Read the model definition and answer for the solid it produces. Units are mm, in the model's axes. Face numbers are marked on the shaded views. A direction names the side the tool comes from. Round coordinates to 2 decimals unless told otherwise and drop trailing zeros. Order: outer loops, then holes, each group sorted by start corner. A loop starts at its lowest first (then second) coordinate and runs counter-clockwise, first axis right, second up.
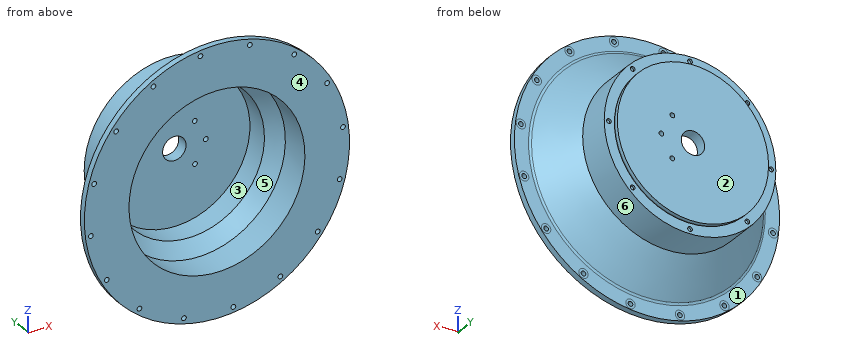
from build123d import *
from build123d.topology import SkipClean

# Parameters (mm, degrees)
SKETCH_1_R               = 85
EXTRUDE_1_DEPTH          = 4
SKETCH_2_R               = 56.4
CUT_EXTRUDE_1_DEPTH      = 50
EXTRUDE_2_REACH          = 125.657
SKETCH_8_R               = 68.956948121
SKETCH_8_R_2             = 56.4
SKETCH_9_R               = 1.5
CUT_EXTRUDE_3_DEPTH      = 5000
PATTERN_CIRCULAR_1_COUNT = 16
SKETCH_11_R              = 52.5
SKETCH_11_R_2            = 48.463912786
EXTRUDE_3_DEPTH          = 30
SKETCH_12_R              = 52.5
SKETCH_12_R_2            = 22.5
EXTRUDE_4_DEPTH          = 5
FILLET_1_R               = 2
SKETCH_13_R              = 85
SKETCH_13_R_2            = 56.4
EXTRUDE_5_DEPTH          = 1
SKETCH_14_R              = 1.5
CUT_EXTRUDE_4_DEPTH      = 50
PATTERN_CIRCULAR_2_COUNT = 16
CHAMFER_2_SIZE           = 5
SKETCH_15_R              = 45
SKETCH_15_R_2            = 43
CUT_EXTRUDE_5_DEPTH      = 2
EXTRUDE_START            = -5
SKETCH_16_R              = 22.5
SKETCH_16_R_2            = 15
EXTRUDE_6_DEPTH          = 5
SKETCH_18_R              = 3
CUT_EXTRUDE_7_DEPTH      = 0.002
PATTERN_CIRCULAR_3_COUNT = 16
EXTRUDE_7_REACH          = 138.657
SKETCH_19_R              = 55
SKETCH_19_R_2            = 49.128121992
SKETCH_20_R              = 47.909164775
SKETCH_20_R_2            = 36.467922282
EXTRUDE_9_DEPTH          = 2
SKETCH_21_R              = 61.010488539
CUT_EXTRUDE_8_DEPTH      = 15
SKETCH_22_R              = 55
EXTRUDE_11_DEPTH         = 5
SKETCH_23_R              = 1.5
CUT_EXTRUDE_9_DEPTH      = 2
PATTERN_CIRCULAR_4_COUNT = 8
SKETCH_24_R              = 48.5
EXTRUDE_12_DEPTH         = 3
SKETCH_25_R              = 7.5
CUT_EXTRUDE_10_DEPTH     = 500
SKETCH_26_R              = 99.377055334
CUT_EXTRUDE_11_DEPTH     = 1
SKETCH_27_R              = 55
SKETCH_27_R_2            = 48.5
CUT_EXTRUDE_13_DEPTH     = 0.5
SKETCH_28_R              = 50.330006294
CUT_EXTRUDE_14_DEPTH     = 0.5
SKETCH_17_R              = 1.5
CUT_EXTRUDE_17_DEPTH     = 20


with BuildPart() as part:
    # 草图1 → 凸台-拉伸1 (new body)
    with BuildSketch(Plane(origin=(0, 0, 0), x_dir=(1, 0, 0), z_dir=(0, 1, 0))):
        with Locations(Location((0, 0, 0), (0, 0, 270))):
            Circle(SKETCH_1_R)
    extrude(amount=EXTRUDE_1_DEPTH)

    # 草图2 → 切除-拉伸1 (cut)
    with BuildSketch(Plane(origin=(0, 4, 0), x_dir=(1, 0, 0), z_dir=(0, 1, 0))):
        with Locations(Location((0, 0, 0), (0, 0, 270))):
            Circle(SKETCH_2_R)
    extrude(amount=-CUT_EXTRUDE_1_DEPTH, mode=Mode.SUBTRACT)

    # 草图3 → 旋转1 (revolve)
    with BuildSketch(Plane.XY):
        Polygon((0, 4), (-75, 4), (-52.5, 29), (0, 29), align=None)
    revolve(axis=Axis((0, 29, 0), (0, -1, 0)))

    # 草图7 → 切除-旋转1 (revolve, cut)
    with BuildSketch(Plane.XY, mode=Mode.PRIVATE) as cut_revolve_1_sk:
        Polygon((0, 4), (-70.963912786, 4), (-48.463912786, 29), (0, 29), align=None)
    revolve(cut_revolve_1_sk.sketch.rotate(Axis((0, 29, 0), (0, -1, 0)), 270), axis=Axis((0, 29, 0), (0, -1, 0)), mode=Mode.SUBTRACT)

    # 凸台-拉伸2: up to this cone (the profile starts inside it)
    extrude_2_end = Plane(origin=(0, 0, 0), z_dir=(0, -1, 0)).offset(-82.848790984) * Cone(1e-06, 255.212734293, 283.56970377, align=(Align.CENTER, Align.CENTER, Align.MIN), mode=Mode.PRIVATE)
    # 草图8 → 凸台-拉伸2 (add, up to the surface)
    with BuildSketch(Plane.XZ, mode=Mode.PRIVATE) as extrude_2_sk1:
        with Locations(Location((0, 0, 0), (0, 0, 270))):
            Circle(SKETCH_8_R)
        with Locations(Location((0, 0, 0), (0, 0, 90))):
            Circle(SKETCH_8_R_2, mode=Mode.SUBTRACT)
    extrude_2_tool1 = extrude(extrude_2_sk1.sketch, amount=-EXTRUDE_2_REACH, mode=Mode.PRIVATE) & extrude_2_end
    add(extrude_2_tool1.solids().sort_by_distance((0, 0, 67.006551))[0])

    # 草图9 → 切除-拉伸3 (cut)
    with BuildSketch(Plane(origin=(0, 4, 0), x_dir=(1, 0, 0), z_dir=(0, 1, 0))):
        with Locations(Location((-40.694024124, -70.613358514, 0), (0, 0, 270))):
            Circle(SKETCH_9_R)
    cut_extrude_3 = extrude(amount=-CUT_EXTRUDE_3_DEPTH, mode=Mode.SUBTRACT)

    # 阵列(圆周)1: 切除-拉伸3 ×16 about axis
    pattern_circular_1_axis = Axis((0, 0, 0), (0, 1, 0))
    for i in range(1, PATTERN_CIRCULAR_1_COUNT):
        add(cut_extrude_3.rotate(pattern_circular_1_axis, i * 360 / PATTERN_CIRCULAR_1_COUNT), mode=Mode.SUBTRACT)

    # 草图11 → 凸台-拉伸3 (add)
    with BuildSketch(Plane(origin=(0, 29, 0), x_dir=(1, 0, 0), z_dir=(0, 1, 0))):
        with Locations(Location((0, 0, 0), (0, 0, 180))):
            Circle(SKETCH_11_R)
        with Locations(Location((0, 0, 0), (0, 0, 180))):
            Circle(SKETCH_11_R_2, mode=Mode.SUBTRACT)
    extrude(amount=EXTRUDE_3_DEPTH)

    # 草图12 → 凸台-拉伸4 (add)
    with BuildSketch(Plane(origin=(0, 59, 0), x_dir=(1, 0, 0), z_dir=(0, 1, 0))):
        with Locations(Location((0, 0, 0), (0, 0, 180))):
            Circle(SKETCH_12_R)
        with Locations(Location((0, 0, 0), (0, 0, 180))):
            Circle(SKETCH_12_R_2, mode=Mode.SUBTRACT)
    extrude(amount=EXTRUDE_4_DEPTH)

    # 圆角1
    fillet_1_edges = [part.edges().sort_by_distance(p)[0] for p in [
        (75, 4, 0),
    ]]
    fillet(fillet_1_edges, radius=FILLET_1_R)

    # 草图13 → 凸台-拉伸5 (add)
    with SkipClean():  # the faces are left unmerged after this step: merging them gives an invalid solid
        with BuildSketch(Plane.XZ):
            with Locations(Location((0, 0, 0), (0, 0, 270))):
                Circle(SKETCH_13_R)
            with Locations(Location((0, 0, 0), (0, 0, 270))):
                Circle(SKETCH_13_R_2, mode=Mode.SUBTRACT)
        extrude(amount=EXTRUDE_5_DEPTH)

    # 草图14 → 切除-拉伸4 (cut)
    with SkipClean():  # the faces are left unmerged after this step: merging them gives an invalid solid
        with BuildSketch(Plane(origin=(0, 4, 0), x_dir=(1, 0, 0), z_dir=(0, 1, 0))):
            with Locations(Location((-70.613358514, 40.694024124, 0), (0, 0, 180))):
                Circle(SKETCH_14_R)
        cut_extrude_4 = extrude(amount=-CUT_EXTRUDE_4_DEPTH, mode=Mode.SUBTRACT)

    # 阵列(圆周)2: 切除-拉伸4 ×16 about axis
    with SkipClean():  # the faces are left unmerged after this step: merging them gives an invalid solid
        pattern_circular_2_axis = Axis((0, 0, 0), (0, 1, 0))
        for i in range(1, PATTERN_CIRCULAR_2_COUNT):
            add(cut_extrude_4.rotate(pattern_circular_2_axis, i * 360 / PATTERN_CIRCULAR_2_COUNT), mode=Mode.SUBTRACT)

    # 倒角2
    chamfer_2_edges = [part.edges().sort_by_distance(p)[0] for p in [
        (48.463912786, 59, 0),
    ]]
    chamfer(chamfer_2_edges, length=CHAMFER_2_SIZE)

    # 草图15 → 切除-拉伸5 (cut)
    with SkipClean():  # the faces are left unmerged after this step: merging them gives an invalid solid
        with BuildSketch(Plane(origin=(0, 64, 0), x_dir=(1, 0, 0), z_dir=(0, 1, 0))):
            with Locations(Location((0, 0, 0), (0, 0, 180))):
                Circle(SKETCH_15_R)
            with Locations(Location((0, 0, 0), (0, 0, 180))):
                Circle(SKETCH_15_R_2, mode=Mode.SUBTRACT)
        extrude(amount=-CUT_EXTRUDE_5_DEPTH, mode=Mode.SUBTRACT)

    # 草图16 → 凸台-拉伸6 (add)
    with SkipClean():  # the faces are left unmerged after this step: merging them gives an invalid solid
        with BuildSketch(Plane(origin=(0, 64, 0), x_dir=(1, 0, 0), z_dir=(0, 1, 0)).offset(EXTRUDE_START)):
            Circle(SKETCH_16_R)
            with Locations(Location((0, 0, 0), (0, 0, 180))):
                Circle(SKETCH_16_R_2, mode=Mode.SUBTRACT)
        extrude(amount=EXTRUDE_6_DEPTH)

    # 草图18 → 切除-拉伸7 (cut)
    with SkipClean():  # the faces are left unmerged after this step: merging them gives an invalid solid
        with BuildSketch(Plane(origin=(0, 4, 0), x_dir=(1, 0, 0), z_dir=(0, 1, 0))):
            with Locations(Location((-80.811165481, 10.573813577, 0), (0, 0, 270))):
                Circle(SKETCH_18_R)
        cut_extrude_7 = extrude(amount=-CUT_EXTRUDE_7_DEPTH, mode=Mode.SUBTRACT)

    # 阵列(圆周)3: 切除-拉伸7 ×16 about axis
    with SkipClean():  # the faces are left unmerged after this step: merging them gives an invalid solid
        pattern_circular_3_axis = Axis((0, 0, 0), (0, 1, 0))
        for i in range(1, PATTERN_CIRCULAR_3_COUNT):
            add(cut_extrude_7.rotate(pattern_circular_3_axis, i * 360 / PATTERN_CIRCULAR_3_COUNT), mode=Mode.SUBTRACT)

    # 凸台-拉伸7: up to this cone (the profile starts outside it)
    with SkipClean():  # the faces are left unmerged after this step: merging them gives an invalid solid
        extrude_7_end = Plane(origin=(0, 64, 0), z_dir=(0, -1, 0)).offset(-23.333332333) * Cone(1e-06, 165.1413, 183.490332333, align=(Align.CENTER, Align.CENTER, Align.MIN), mode=Mode.PRIVATE)
        # 草图19 → 凸台-拉伸7 (add, up to the surface)
        with BuildSketch(Plane(origin=(0, 64, 0), x_dir=(1, 0, 0), z_dir=(0, 1, 0)), mode=Mode.PRIVATE) as extrude_7_sk1:
            with Locations(Location((0, 0, 0), (0, 0, 180))):
                Circle(SKETCH_19_R)
            Circle(SKETCH_19_R_2, mode=Mode.SUBTRACT)
        extrude_7_tool1 = extrude(extrude_7_sk1.sketch, amount=-EXTRUDE_7_REACH, mode=Mode.PRIVATE) - extrude_7_end
        add(extrude_7_tool1.solids().sort_by_distance((53.444365, 64, 0))[0])

    # 草图20 → 凸台-拉伸9 (add)
    with SkipClean():  # the faces are left unmerged after this step: merging them gives an invalid solid
        with BuildSketch(Plane(origin=(0, 64, 0), x_dir=(1, 0, 0), z_dir=(0, 1, 0))):
            Circle(SKETCH_20_R)
            Circle(SKETCH_20_R_2, mode=Mode.SUBTRACT)
        extrude(amount=-EXTRUDE_9_DEPTH)

    # 草图21 → 切除-拉伸8 (cut)
    with SkipClean():  # the faces are left unmerged after this step: merging them gives an invalid solid
        with BuildSketch(Plane(origin=(0, 64, 0), x_dir=(1, 0, 0), z_dir=(0, 1, 0))):
            Circle(SKETCH_21_R)
        extrude(amount=-CUT_EXTRUDE_8_DEPTH, mode=Mode.SUBTRACT)

    # 草图22 → 凸台-拉伸11 (add)
    with SkipClean():  # the faces are left unmerged after this step: merging them gives an invalid solid
        with BuildSketch(Plane(origin=(0, 49, 0), x_dir=(1, 0, 0), z_dir=(0, 1, 0))):
            with Locations(Location((0, 0, 0), (0, 0, 180))):
                Circle(SKETCH_22_R)
        extrude(amount=-EXTRUDE_11_DEPTH)

    # 草图23 → 切除-拉伸9 (cut)
    with SkipClean():  # the faces are left unmerged after this step: merging them gives an invalid solid
        with BuildSketch(Plane(origin=(0, 49, 0), x_dir=(1, 0, 0), z_dir=(0, 1, 0))):
            with Locations(Location((52, 0, 0), (0, 0, 180))):
                Circle(SKETCH_23_R)
        cut_extrude_9 = extrude(amount=-CUT_EXTRUDE_9_DEPTH, mode=Mode.SUBTRACT)

    # 阵列(圆周)4: 切除-拉伸9 ×8 about axis
    with SkipClean():  # the faces are left unmerged after this step: merging them gives an invalid solid
        pattern_circular_4_axis = Axis((0, 0, 0), (0, 1, 0))
        for i in range(1, PATTERN_CIRCULAR_4_COUNT):
            add(cut_extrude_9.rotate(pattern_circular_4_axis, i * 360 / PATTERN_CIRCULAR_4_COUNT), mode=Mode.SUBTRACT)

    # 草图24 → 凸台-拉伸12 (add)
    with SkipClean():  # the faces are left unmerged after this step: merging them gives an invalid solid
        with BuildSketch(Plane(origin=(0, 49, 0), x_dir=(1, 0, 0), z_dir=(0, 1, 0))):
            with Locations(Location((0, 0, 0), (0, 0, 180))):
                Circle(SKETCH_24_R)
        extrude(amount=EXTRUDE_12_DEPTH)

    # 草图25 → 切除-拉伸10 (cut)
    with SkipClean():  # the faces are left unmerged after this step: merging them gives an invalid solid
        with BuildSketch(Plane(origin=(0, 52, 0), x_dir=(1, 0, 0), z_dir=(0, 1, 0))):
            with Locations(Location((0, 0, 0), (0, 0, 180))):
                Circle(SKETCH_25_R)
        extrude(amount=-CUT_EXTRUDE_10_DEPTH, mode=Mode.SUBTRACT)

    # 草图26 → 切除-拉伸11 (cut)
    with BuildSketch(Plane.XZ.offset(1)):
        Circle(SKETCH_26_R)
    extrude(amount=-CUT_EXTRUDE_11_DEPTH, mode=Mode.SUBTRACT)

    # 草图27 → 切除-拉伸13 (cut)
    with BuildSketch(Plane(origin=(0, 49, 0), x_dir=(1, 0, 0), z_dir=(0, 1, 0))):
        with Locations(Location((0, 0, 0), (0, 0, 180))):
            Circle(SKETCH_27_R)
        with Locations(Location((0, 0, 0), (0, 0, 180))):
            Circle(SKETCH_27_R_2, mode=Mode.SUBTRACT)
    extrude(amount=-CUT_EXTRUDE_13_DEPTH, mode=Mode.SUBTRACT)

    # 草图28 → 切除-拉伸14 (cut)
    with BuildSketch(Plane(origin=(0, 52, 0), x_dir=(1, 0, 0), z_dir=(0, 1, 0))):
        Circle(SKETCH_28_R)
    extrude(amount=-CUT_EXTRUDE_14_DEPTH, mode=Mode.SUBTRACT)

    # 草图17 → 切除-拉伸17 (cut)
    with BuildSketch(Plane(origin=(0, 64, 0), x_dir=(1, 0, 0), z_dir=(0, 1, 0))):
        with Locations(Location((13.161077513, -13.427494448, 0), (0, 0, 180))):
            Circle(SKETCH_17_R)
        with Locations(Location((20.214261652, -0.080464123, 0), (0, 0, 180))):
            Circle(SKETCH_17_R)
        with Locations(Location((13.267556705, 13.322293629, 0), (0, 0, 180))):
            Circle(SKETCH_17_R)
    extrude(amount=-CUT_EXTRUDE_17_DEPTH, mode=Mode.SUBTRACT)


solid = part.part
Q1. For the marked faces 1, 2 and 3, determine the directions among +Z, -Z, +X, -X, +Y, -Y from which every point of the face is accessible in a straight line to the end or side of a thin tool.
Outcome:
face 1: +Y
face 2: +Z, -Z, +X, -X, +Y
face 3: -Y
Q2. Straight lines are drawn through the part: probe 1 along Z at (x, y) = (60, 6); probe 2 along X at (y, z) = (9, 44); probe 3 along Y at (x, z) = (-30.5, -11). For each, find the intervals that lie inside material, in ascending order.
Outcome:
probe 1: z = -41.93 to -34.4, -33.99 to 33.99, 34.4 to 41.93
probe 2: x = -55.08 to -35.28, 35.28 to 55.08
probe 3: y = 44 to 51.5
Q3. A cutting plane is placed at A-A, the plane y = 36.5. Give the vertices of the cut face in (x, z).
Outcome:
outline: circle Ø110 at (0, 0); hole circle Ø96.93 at (0, 0)
Q4. For a pull along Z with two mould halves and no side action, classify the marked faces 4, 5 and 6 as released by +Z, released by -Z, zero draft, split by the parting line, or undercut.
Outcome:
face 4: zero draft
face 5: undercut
face 6: split by the parting line
Q5. A cutting plane is placed at B-B, the plane y = 10. Give the vertices of the cut face in (x, z), plus the area to 3 significant figures.
Outcome:
outline: circle Ø139.2 at (0, 0); hole circle Ø112.8 at (0, 0)
area: 5,230 mm2
Q6. Flat-ended cylindrical pins translate along their axes: pin 1 (3 mm diameter, centred on x = -22, z = -78, fed in from +Y); pin 2 (1 mm diameter, centred on y = 41, z = 5.5, fed in from +X); pin 3 (2.5 mm diameter, centred on x = 0, z = 52, fed in from +Y); pin 4 (2.5 mm diameter, centred on x = 49.67, z = 64.62, fed in from +Y). Find the tip coordinate at first contact, or state that the pin passes through.
Outcome:
pin 1: stops at y = 4
pin 2: stops at x = 54.77
pin 3: stops at y = 47
pin 4: passes through
